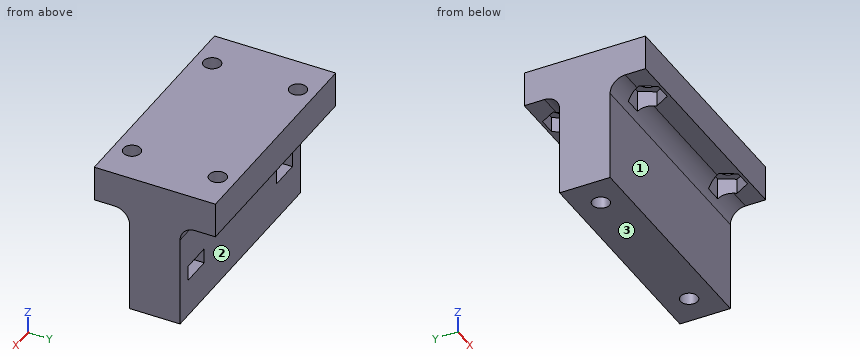
```python
from build123d import *

# Parameters (mm, degrees)
SKETCH_1_W          = 45
SKETCH_1_H          = 20
EXTRUDE_1_DEPTH     = 10
EXTRUDE_2_DEPTH     = 17
SKETCH_3_W          = 45
SKETCH_3_H          = 2
EXTRUDE_3_DEPTH     = 10
SKETCH_5_R          = 1.5
CUT_EXTRUDE_1_DEPTH = 31.647185841
CUT_EXTRUDE_3_DEPTH = 3
FILLET_4_R          = 3
FILLET_5_R          = 3
SKETCH_9_W          = 45
SKETCH_9_H          = 24
CUT_EXTRUDE_4_DEPTH = 3
SKETCH_10_W         = 45
SKETCH_10_H         = 10
EXTRUDE_4_DEPTH     = 3
SKETCH_12_R         = 1.55
CUT_EXTRUDE_5_DEPTH = 15
CUT_EXTRUDE_6_DEPTH = 8
EXTRUDE_START       = 1
SKETCH_15_W         = 45
SKETCH_15_H         = 10
SKETCH_15_R         = 1.55
EXTRUDE_5_DEPTH     = 1
SKETCH_16_R         = 1.7
CUT_EXTRUDE_7_DEPTH = 38.871493237
CUT_EXTRUDE_8_DEPTH = 24
CUT_EXTRUDE_9_REACH = 39.871
SKETCH_18_R         = 1.7


with BuildPart() as part:
    # Эскиз1 → Бобышка-Вытянуть1 (new body)
    with BuildSketch(Plane.XY):
        Rectangle(SKETCH_1_W, SKETCH_1_H)
    extrude(amount=EXTRUDE_1_DEPTH)

    # Эскиз2 → Бобышка-Вытянуть2 (add)
    with BuildSketch(Plane(origin=(0, 0, 0), x_dir=(-1, 0, 0), z_dir=(0, 0, -1))):
        Polygon((-22.5, 0), (-22.5, 5), (22.5, 5), (22.5, -5), (-22.5, -5), align=None)
    extrude(amount=EXTRUDE_2_DEPTH)

    # Эскиз3 → Бобышка-Вытянуть3 (add)
    with BuildSketch(Plane.XY.offset(10)):
        with Locations((0, 11)):
            Rectangle(SKETCH_3_W, SKETCH_3_H)
        with Locations((0, -11)):
            Rectangle(SKETCH_3_W, SKETCH_3_H)
    extrude(amount=-EXTRUDE_3_DEPTH)

    # Эскиз5 → Вырез-Вытянуть1 (cut, through all)
    with BuildSketch(Plane(origin=(0, 0, 0), x_dir=(-1, 0, 0), z_dir=(0, 0, -1))):
        with Locations((-15, 8.5)):
            Circle(SKETCH_5_R)
        with Locations((15, 8.5)):
            Circle(SKETCH_5_R)
        with Locations((15, -8.5)):
            Circle(SKETCH_5_R)
        with Locations((-15, -8.5)):
            Circle(SKETCH_5_R)
    extrude(amount=-CUT_EXTRUDE_1_DEPTH, mode=Mode.SUBTRACT)

    # Эскиз8 → Вырез-Вытянуть3 (cut)
    with BuildSketch(Plane(origin=(0, 0, 0), x_dir=(-1, 0, 0), z_dir=(0, 0, -1))):
        Polygon((-11.824573519, 8.5), (-13.41228676, 11.25), (-16.58771324, 11.25), (-18.175426481, 8.5), (-16.58771324, 5.75), (-13.41228676, 5.75), align=None)
        Polygon((-13.41228676, -5.75), (-11.824573519, -8.5), (-13.41228676, -11.25), (-16.58771324, -11.25), (-18.175426481, -8.5), (-16.58771324, -5.75), align=None)
        Polygon((11.824573519, -8.5), (13.41228676, -11.25), (16.58771324, -11.25), (18.175426481, -8.5), (16.58771324, -5.75), (13.41228676, -5.75), align=None)
        Polygon((13.41228676, 5.75), (11.824573519, 8.5), (13.41228676, 11.25), (16.58771324, 11.25), (18.175426481, 8.5), (16.58771324, 5.75), align=None)
    extrude(amount=-CUT_EXTRUDE_3_DEPTH, mode=Mode.SUBTRACT)

    # Скругление4
    # the kernel refuses this fillet: 3 mm, written as the material it adds along each edge
    with BuildSketch(Plane(origin=(22.5, 5, 0), x_dir=(0, 1, 0), z_dir=(-1, 0, 0))) as fillet_4_piece_1_section:
        with BuildLine():
            CenterArc((FILLET_4_R, FILLET_4_R), FILLET_4_R, 180, 90)
            Line((0, FILLET_4_R), (0, 0))
            Line((0, 0), (FILLET_4_R, 0))
        make_face()
    fillet_4_piece_1 = extrude(amount=52.5, mode=Mode.PRIVATE)
    fillet_4_piece_1 = split(fillet_4_piece_1, bisect_by=Plane(origin=(17.590792641, 7.487384486, -0.29904688), z_dir=(0.866025403784439, -0.49999999999999944, 0)), keep=Keep.TOP, mode=Mode.PRIVATE)
    add(fillet_4_piece_1)
    with BuildSketch(Plane(origin=(30, 5, 0), x_dir=(0, 1, 0), z_dir=(-1, 0, 0))) as fillet_4_piece_2_section:
        with BuildLine():
            CenterArc((FILLET_4_R, FILLET_4_R), FILLET_4_R, 180, 90)
            Line((0, FILLET_4_R), (0, 0))
            Line((0, 0), (FILLET_4_R, 0))
        make_face()
    fillet_4_piece_2 = extrude(amount=52.5, mode=Mode.PRIVATE)
    fillet_4_piece_2 = split(fillet_4_piece_2, bisect_by=Plane(origin=(16.011289033, 4.751603986, -0.863215568), z_dir=(-0.866025403784439, 0.49999999999999944, 0)), keep=Keep.TOP, mode=Mode.PRIVATE)
    fillet_4_piece_2 = split(fillet_4_piece_2, bisect_by=Plane(origin=(15, 5.75, -0.863215568), z_dir=(0, -1, 0)), keep=Keep.TOP, mode=Mode.PRIVATE)
    add(fillet_4_piece_2)
    with BuildSketch(Plane(origin=(30, 5, 0), x_dir=(0, 1, 0), z_dir=(-1, 0, 0))) as fillet_4_piece_3_section:
        with BuildLine():
            CenterArc((FILLET_4_R, FILLET_4_R), FILLET_4_R, 180, 90)
            Line((0, FILLET_4_R), (0, 0))
            Line((0, 0), (FILLET_4_R, 0))
        make_face()
    fillet_4_piece_3 = extrude(amount=60, mode=Mode.PRIVATE)
    fillet_4_piece_3 = split(fillet_4_piece_3, bisect_by=Plane(origin=(9.828179478, 11.957855912, -0.295719997), z_dir=(-0.8660254037844385, -0.5000000000000003, 0)), keep=Keep.TOP, mode=Mode.PRIVATE)
    fillet_4_piece_3 = split(fillet_4_piece_3, bisect_by=Plane(origin=(-9.828179478, 11.957855912, -0.295719997), z_dir=(0.8660254037844385, -0.5000000000000003, 0)), keep=Keep.TOP, mode=Mode.PRIVATE)
    add(fillet_4_piece_3)
    with BuildSketch(Plane(origin=(30, 5, 0), x_dir=(0, 1, 0), z_dir=(-1, 0, 0))) as fillet_4_piece_4_section:
        with BuildLine():
            CenterArc((FILLET_4_R, FILLET_4_R), FILLET_4_R, 180, 90)
            Line((0, FILLET_4_R), (0, 0))
            Line((0, 0), (FILLET_4_R, 0))
        make_face()
    fillet_4_piece_4 = extrude(amount=52.5, mode=Mode.PRIVATE)
    fillet_4_piece_4 = split(fillet_4_piece_4, bisect_by=Plane(origin=(-17.590792641, 7.487384486, -0.29904688), z_dir=(-0.866025403784439, -0.49999999999999944, 0)), keep=Keep.TOP, mode=Mode.PRIVATE)
    add(fillet_4_piece_4)

    # Скругление5
    # the kernel refuses this fillet: 3 mm, written as the material it adds along each edge
    with BuildSketch(Plane(origin=(-22.5, -5, 0), x_dir=(0, 0, -1), z_dir=(1, 0, 0))) as fillet_5_piece_1_section:
        with BuildLine():
            CenterArc((FILLET_5_R, -FILLET_5_R), FILLET_5_R, 90, 90)
            Line((0, -FILLET_5_R), (0, 0))
            Line((0, 0), (FILLET_5_R, 0))
        make_face()
    fillet_5_piece_1 = extrude(amount=45, mode=Mode.PRIVATE)
    fillet_5_piece_1 = split(fillet_5_piece_1, bisect_by=Plane(origin=(-19.417241341, -5.75, -0.889716038), z_dir=(0, 1, 0)), keep=Keep.TOP, mode=Mode.PRIVATE)
    add(fillet_5_piece_1)
    with BuildSketch(Plane(origin=(-22.5, -5, 0), x_dir=(0, 0, -1), z_dir=(1, 0, 0))) as fillet_5_piece_2_section:
        with BuildLine():
            CenterArc((FILLET_5_R, -FILLET_5_R), FILLET_5_R, 90, 90)
            Line((0, -FILLET_5_R), (0, 0))
            Line((0, 0), (FILLET_5_R, 0))
        make_face()
    fillet_5_piece_2 = extrude(amount=52.5, mode=Mode.PRIVATE)
    fillet_5_piece_2 = split(fillet_5_piece_2, bisect_by=Plane(origin=(-17.590792641, -7.487384486, -0.29904688), z_dir=(-0.866025403784439, 0.49999999999999944, 0)), keep=Keep.TOP, mode=Mode.PRIVATE)
    add(fillet_5_piece_2)
    with BuildSketch(Plane(origin=(-30, -5, 0), x_dir=(0, 0, -1), z_dir=(1, 0, 0))) as fillet_5_piece_3_section:
        with BuildLine():
            CenterArc((FILLET_5_R, -FILLET_5_R), FILLET_5_R, 90, 90)
            Line((0, -FILLET_5_R), (0, 0))
            Line((0, 0), (FILLET_5_R, 0))
        make_face()
    fillet_5_piece_3 = extrude(amount=60, mode=Mode.PRIVATE)
    fillet_5_piece_3 = split(fillet_5_piece_3, bisect_by=Plane(origin=(-9.828179478, -11.957855912, -0.295719997), z_dir=(0.8660254037844385, 0.5000000000000003, 0)), keep=Keep.TOP, mode=Mode.PRIVATE)
    fillet_5_piece_3 = split(fillet_5_piece_3, bisect_by=Plane(origin=(9.828179478, -11.957855912, -0.295719997), z_dir=(-0.8660254037844385, 0.5000000000000003, 0)), keep=Keep.TOP, mode=Mode.PRIVATE)
    add(fillet_5_piece_3)
    with BuildSketch(Plane(origin=(-30, -5, 0), x_dir=(0, 0, -1), z_dir=(1, 0, 0))) as fillet_5_piece_4_section:
        with BuildLine():
            CenterArc((FILLET_5_R, -FILLET_5_R), FILLET_5_R, 90, 90)
            Line((0, -FILLET_5_R), (0, 0))
            Line((0, 0), (FILLET_5_R, 0))
        make_face()
    fillet_5_piece_4 = extrude(amount=52.5, mode=Mode.PRIVATE)
    fillet_5_piece_4 = split(fillet_5_piece_4, bisect_by=Plane(origin=(17.590792641, -7.487384486, -0.29904688), z_dir=(0.866025403784439, 0.49999999999999944, 0)), keep=Keep.TOP, mode=Mode.PRIVATE)
    add(fillet_5_piece_4)

    # Эскиз9 → Вырез-Вытянуть4 (cut)
    with BuildSketch(Plane.XY.offset(10)):
        Rectangle(SKETCH_9_W, SKETCH_9_H)
    extrude(amount=-CUT_EXTRUDE_4_DEPTH, mode=Mode.SUBTRACT)

    # Эскиз10 → Бобышка-Вытянуть4 (add)
    with BuildSketch(Plane(origin=(0, 0, -17), x_dir=(-1, 0, 0), z_dir=(0, 0, -1))):
        Rectangle(SKETCH_10_W, SKETCH_10_H)
    extrude(amount=EXTRUDE_4_DEPTH)

    # Эскиз12 → Вырез-Вытянуть5 (cut)
    with BuildSketch(Plane(origin=(0, 0, -20), x_dir=(-1, 0, 0), z_dir=(0, 0, -1))):
        with Locations((-16.5, 0)):
            Circle(SKETCH_12_R)
        with Locations((16.5, 0)):
            Circle(SKETCH_12_R)
    extrude(amount=-CUT_EXTRUDE_5_DEPTH, mode=Mode.SUBTRACT)

    # Эскиз13 → Вырез-Вытянуть6 (cut)
    with BuildSketch(Plane(origin=(0, 5, 0), x_dir=(1, 0, 0), z_dir=(0, 1, 0))):
        Polygon((16.5, 13.5), (13.5, 13.5), (13.5, 10.5), (19.5, 10.5), (19.5, 13.5), align=None)
        Polygon((-19.5, 13.5), (-16.5, 13.5), (-13.5, 13.5), (-13.5, 10.5), (-19.5, 10.5), align=None)
    extrude(amount=-CUT_EXTRUDE_6_DEPTH, mode=Mode.SUBTRACT)

    # Эскиз15 → Бобышка-Вытянуть5 (add)
    with BuildSketch(Plane(origin=(0, 0, -20), x_dir=(-1, 0, 0), z_dir=(0, 0, -1)).offset(EXTRUDE_START)):
        Rectangle(SKETCH_15_W, SKETCH_15_H)
        with Locations((-16.5, 0)):
            Circle(SKETCH_15_R, mode=Mode.SUBTRACT)
        with Locations((16.5, 0)):
            Circle(SKETCH_15_R, mode=Mode.SUBTRACT)
    extrude(amount=-EXTRUDE_5_DEPTH)

    # Эскиз16 → Вырез-Вытянуть7 (cut, through all)
    with BuildSketch(Plane.XY.offset(7)):
        with Locations((15, -8.5)):
            Circle(SKETCH_16_R)
        with Locations((-15, -8.5)):
            Circle(SKETCH_16_R)
        with Locations((-15, 8.5)):
            Circle(SKETCH_16_R)
        with Locations((15, 8.5)):
            Circle(SKETCH_16_R)
    extrude(amount=-CUT_EXTRUDE_7_DEPTH, mode=Mode.SUBTRACT)

    # Эскиз17 → Вырез-Вытянуть8 (cut)
    with BuildSketch(Plane(origin=(0, 0, -21), x_dir=(-1, 0, 0), z_dir=(0, 0, -1))):
        Polygon((-13.296816706, 5.55), (-11.593633412, 8.5), (-13.296816706, 11.45), (-16.703183294, 11.45), (-18.406366588, 8.5), (-16.703183294, 5.55), align=None)
        Polygon((16.703183294, 5.55), (18.406366588, 8.5), (16.703183294, 11.45), (13.296816706, 11.45), (11.593633412, 8.5), (13.296816706, 5.55), align=None)
        Polygon((16.703183294, -11.45), (18.406366588, -8.5), (16.703183294, -5.55), (13.296816706, -5.55), (11.593633412, -8.5), (13.296816706, -11.45), align=None)
        Polygon((-13.296816706, -11.45), (-11.593633412, -8.5), (-13.296816706, -5.55), (-16.703183294, -5.55), (-18.406366588, -8.5), (-16.703183294, -11.45), align=None)
    extrude(amount=-CUT_EXTRUDE_8_DEPTH, mode=Mode.SUBTRACT)

    # Вырез-Вытянуть9: up to this face of the body (flat: up to its plane)
    cut_extrude_9_end = Plane(part.part.faces().sort_by_distance((16.5, 0, -5))[0])
    # Эскиз18 → Вырез-Вытянуть9 (cut, up to the picked face)
    with BuildSketch(Plane(origin=(0, 0, -21), x_dir=(-1, 0, 0), z_dir=(0, 0, -1)), mode=Mode.PRIVATE) as cut_extrude_9_sk1:
        with Locations((-16.5, 0)):
            Circle(SKETCH_18_R)
    cut_extrude_9_tool1 = split(extrude(cut_extrude_9_sk1.sketch, amount=-CUT_EXTRUDE_9_REACH, mode=Mode.PRIVATE), bisect_by=cut_extrude_9_end, keep=Keep.BOTH, mode=Mode.PRIVATE)
    # Эскиз18 → Вырез-Вытянуть9 (cut, up to the picked face)
    with BuildSketch(Plane(origin=(0, 0, -21), x_dir=(-1, 0, 0), z_dir=(0, 0, -1)), mode=Mode.PRIVATE) as cut_extrude_9_sk2:
        with Locations((16.5, 0)):
            Circle(SKETCH_18_R)
    cut_extrude_9_tool2 = split(extrude(cut_extrude_9_sk2.sketch, amount=-CUT_EXTRUDE_9_REACH, mode=Mode.PRIVATE), bisect_by=cut_extrude_9_end, keep=Keep.BOTH, mode=Mode.PRIVATE)
    add(cut_extrude_9_tool1.solids().sort_by(Axis((16.5, 0, -21), (0, 0, 1)))[0], mode=Mode.SUBTRACT)
    add(cut_extrude_9_tool2.solids().sort_by(Axis((-16.5, 0, -21), (0, 0, 1)))[0], mode=Mode.SUBTRACT)


solid = part.part
```
Read the model definition and answer for the solid it produces. Units are mm, in the model's axes. Face numbers are marked on the shaded views. A direction names the side the tool comes from. Give positions to 0.01 mm unless a question says otherwise; leave off trailing zeros. Order: outer loops, then holes, each group sorted by start corner. A loop starts at its lowest first (then second) coordinate and runs counter-clockwise, first axis right, second up. Notation, with made-up numbers: (41, 74.25) -> (95, 74.25) arc R35 ccw to (95, 111.25) -> close; hole circle Ø1 at (40, 61.25). An arc over 180 degrees is marked (long way). One line per item, written item: value. Start each with the question number.
(1) The part is cut by section C-C (x = -9.5). Determine the outline of the cut face in (y, z).
(2) A tool of negligible diameter and unlimited length cuts with its end or side. For the marked faces 1, 2 and 3, from which of +Z, -Z, +X, -X, +Y, -Y can it reach the whole face along a straight path? Write none if from no direction.
(3) The part is cut by section A-A (x = 17.5). Determine the outline of the cut face in (y, z), and give its area (3 significant figures).
(4) The part is cut by section B-B (y = 0). Determine the outline of the cut face in (x, z).
(5) The part is cut by section D-D (z = -1.75). Determine the outline of the cut face in (x, y).
(6) Straight lines are drawn through the part: L1, parallel to Y at x = 15, z = 4.95; L2, parallel to Z at x = 18.5, y = 2; L3, parallel to X at y = -8.25, z = 5.5. For each, find the intervals that lie inside material, in ascending order.
(7) Flat-ended cylindrical pins translate along their axes: P1, Ø3, axis at x = 14, z = -15.5, coming from the +Y side; P2, Ø1.8, axis at x = 16, y = 0.5, coming from the -Z side; P3, Ø4.5, axis at x = 15, y = -8.5, coming from the +Z side; P4, Ø4.5, axis at x = 15, y = -7.5, coming from the -Z side. Find the tip coordinate at first contact, or state that the pin passes through.
Taken from the geometry:
1. outline: (-12, 0) -> (-8, 0) arc R3 cw to (-5, -3) -> (-5, -21) -> (5, -21) -> (5, -3) arc R3 cw to (8, 0) -> (12, 0) -> (12, 7) -> (-12, 7) -> close
2. face 1: -Z, +X, -X, -Y
2. face 2: -Z, +X, -X, +Y
2. face 3: -Z, +X, -X, +Y, -Y
3. outline: (-12, 0) -> (-10.07, 0) -> (-10.07, 3) -> (-6.93, 3) -> (-6.93, -0.2) arc R3 cw to (-5, -3) -> (-5, -21) -> (-1.37, -21) -> (-1.37, -13.5) -> (-3, -13.5) -> (-3, -10.5) -> (-1.37, -10.5) -> (-1.37, -5) -> (1.37, -5) -> (1.37, -10.5) -> (5, -10.5) -> (5, -3) arc R3 cw to (6.93, -0.2) -> (6.93, 3) -> (10.07, 3) -> (10.07, 0) -> (12, 0) -> (12, 7) -> (-12, 7) -> close; (1.37, -21) -> (5, -21) -> (5, -13.5) -> (1.37, -13.5) -> close
3. area: 303 mm^2
4. outline: (-22.5, -21) -> (-18.2, -21) -> (-18.2, -13.5) -> (-19.5, -13.5) -> (-19.5, -10.5) -> (-18.2, -10.5) -> (-18.2, -5) -> (-14.8, -5) -> (-14.8, -10.5) -> (-13.5, -10.5) -> (-13.5, -13.5) -> (-14.8, -13.5) -> (-14.8, -21) -> (14.8, -21) -> (14.8, -13.5) -> (13.5, -13.5) -> (13.5, -10.5) -> (14.8, -10.5) -> (14.8, -5) -> (18.2, -5) -> (18.2, -10.5) -> (19.5, -10.5) -> (19.5, -13.5) -> (18.2, -13.5) -> (18.2, -21) -> (22.5, -21) -> (22.5, 7) -> (-22.5, 7) -> close
5. outline: (-22.5, -5.27) -> (22.5, -5.27) -> (22.5, 5.27) -> (-22.5, 5.27) -> close
6. L1: -12 to -10.2, -6.8 to 6.8, 10.2 to 12
6. L2: -21 to -13.5, -10.5 to 7
6. L3: -22.5 to -16.68, -13.32 to 13.32, 16.68 to 22.5
7. P1: y = 5
7. P2: z = -5
7. P3: z = 7
7. P4: z = -1.8
